Can you work these out from the drawing? Everything is in mm from the part's minimum corner. A direction names the side the tool comes from. Coordinates: 2 decimals unless noted, no trailing zeros. Loops run counter-clockwise (first coordinate to the right, second up) from the corner with the lowest first, then second, coordinate; pieces in that order, holes last. Notation, with made-up numbers: (19, 35) - (34, 35) arc R36 cw to (34, 70) - close; hole circle Ø3 at (87.25, -33.5). An arc over 180 degrees is marked (long way). Put each result on its own line as item: value. Start each with the question number.
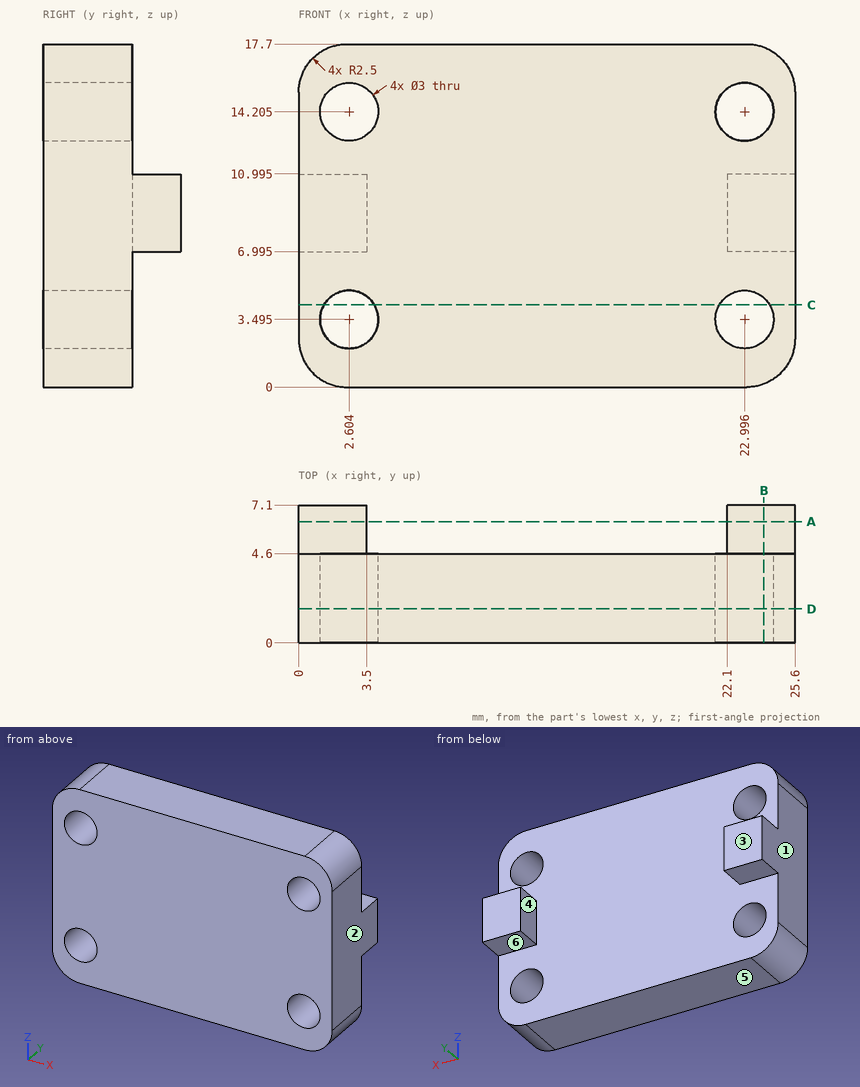
Q1. I want a section at D-D on y = 1.75. List the corners of the cut face in (x, z) for me (1 decimal).
Q2. I want a section at C-C on z = 4.25. List the corners of the cut face in (x, y) for me.
Q3. On a 3-axis mill with a long thin cutter (end or side, diameter ignored), from which of +Z, -Z, +X, -X, +Y, -Y can I reach the whole of each face in a straight line? I mean the marked faces 5 and 6. Say none if no direction works.
Q4. Please list where these lines run through material, in increasing order: line 1 along Z through (x, y) = (23.75, 1.5) (1 decimal); line 2 along Z through (x, y) = (23, 4.5) (1 decimal); line 3 along X through (y, z) = (4, 14.5) (1 decimal). Write a range as [from, to].
Q5. I want a section at B-B on x = 24. List the corners of the cut face in (y, z) for me (1 decimal).
Q6. Will these pins go through, and if not, where does the flat tip stop? pin 1 (10 mm diameter, centred on x = 9, z = 7, fed in from +Y); pin 2 (3 mm diameter, centred on x = 23.5, y = 6.5, fed in from -Z) (1 decimal).
Q7. We'd pull the mould along X, two halves only. Please class the marked faces 1, 2, 3 and 4: released by +X, released by -X, zero draft, split by the parting line, or undercut.
Q8. I want a section at A-A on y = 6.25. List the corners of the cut face in (x, z) for me (1 decimal), and give its area (3 significant figures).
Calculated:
1. outline: (0, 2.5) arc R2.5 ccw to (2.5, 0) - (23.1, 0) arc R2.5 ccw to (25.6, 2.5) - (25.6, 15.2) arc R2.5 ccw to (23.1, 17.7) - (2.5, 17.7) arc R2.5 ccw to (0, 15.2) - close; hole circle Ø3 at (2.6, 3.5); hole circle Ø3 at (2.6, 14.2); hole circle Ø3 at (23, 3.5); hole circle Ø3 at (23, 14.2)
2. outline: (0, 0) - (1.31, 0) - (1.31, 4.6) - (0, 4.6) - close; (3.9, 0) - (21.7, 0) - (21.7, 4.6) - (3.9, 4.6) - close; (24.29, 0) - (25.6, 0) - (25.6, 4.6) - (24.29, 4.6) - close
3. face 5: -Z, +X, -X, +Y, -Y
3. face 6: -Z, +X, -X, +Y
4. line 1: [0.1, 2.2], [4.8, 12.9], [15.5, 17.6]
4. line 2: [0, 2], [5, 12.7], [15.7, 17.7]
4. line 3: [0, 1.1], [4.1, 21.5], [24.5, 25.6]
5. outline: (0, 0.2) - (4.6, 0.2) - (4.6, 2.4) - (0, 2.4) - close; (0, 4.6) - (4.6, 4.6) - (4.6, 7) - (7.1, 7) - (7.1, 11) - (4.6, 11) - (4.6, 13.1) - (0, 13.1) - close; (0, 15.3) - (4.6, 15.3) - (4.6, 17.5) - (0, 17.5) - close
6. pin 1: y = 4.6
6. pin 2: z = 7
7. face 1: released by -X
7. face 2: released by +X
7. face 3: zero draft
7. face 4: undercut
8. outline: (0, 7) - (3.5, 7) - (3.5, 11) - (0, 11) - close; (22.1, 7) - (25.6, 7) - (25.6, 11) - (22.1, 11) - close
8. area: 28.0 mm2
